Check sheet for the modelled part. Datum: model origin and axes. Units: mm. A direction names the side the tool comes from. Give positions to 0.01 mm unless a question says otherwise; leave off trailing zeros. Loops run counter-clockwise (first coordinate to the right, second up) from the corner with the lowest first, then second, coordinate; pieces in that order, holes last. Notation, with made-up numbers: (69.5, 33) - (122.5, 33) arc R23 ccw to (122.5, 61) - close; hole circle Ø9 at (52.25, 34). An arc over 180 degrees is marked (long way). Use one line per item in the form item = value.
from build123d import *

# Parameters (mm, degrees)
F0_R     = 2.25
F0_R_2   = 1
F1_DEPTH = 4


with BuildPart() as f1:
    # F0 (on Front) → F1 (new body)
    with BuildSketch(Plane.XZ):
        with BuildLine():
            ThreePointArc((0.754098, -10), (7.825165, -7.071068), (10.754098, 0))
            Line((10.754098, 0), (10.754098, 10))
            Line((10.754098, 10), (10.754098, 15))
            Line((10.754098, 15), (10.754098, 25))
            ThreePointArc((10.754098, 25), (9.289631, 28.535534), (5.754098, 30))
            ThreePointArc((5.754098, 30), (-1.31697, 27.071068), (-4.245902, 20))
            Line((-4.245902, 20), (-4.245902, 15))
            ThreePointArc((-4.245902, 15), (-5.710369, 11.464466), (-9.245902, 10))
            Line((-9.245902, 10), (-15.348779, 10))
            ThreePointArc((-15.348779, 10), (-25.348779, 0), (-15.348779, -10))
            Line((-15.348779, -10), (0, -10))
            Line((0, -10), (0.754098, -10))
        make_face()
        with Locations((-15.348779, 0)):
            Circle(F0_R, mode=Mode.SUBTRACT)
        Circle(F0_R, mode=Mode.SUBTRACT)
        with Locations((6.754098, 15)):
            Circle(F0_R_2, mode=Mode.SUBTRACT)
        with Locations((6.754098, 25)):
            Circle(F0_R_2, mode=Mode.SUBTRACT)
    extrude(amount=F1_DEPTH)


solid = f1.part
Item 1: Section check B-B on x = -0.5. Record the boundary of the cut face in (y, z).
Answer block:
outline = (-4, -10) - (0, -10) - (0, -2.19) - (-4, -2.19) - close; (-4, 2.19) - (0, 2.19) - (0, 27.8) - (-4, 27.8) - close
Item 2: Gauge pin test, flat ends, axial feed: P1, Ø1.6, axis at x = 6.75, z = 15, coming from the +Y side; P2, Ø2.5, axis at x = 6.75, z = 25, coming from the +Y side; P3, Ø1.2, axis at x = -11, y = -2, coming from the +Z side. Record the tip position at first contact, or that the pin passes through.
Answer block:
P1 = through
P2 = 0
P3 = 10
Item 3: Thickness scan on L1, parallel to X at y = -0.9, z = 17; L2, parallel to Z at x = -12.5, y = -0.4; L3, parallel to Z at x = 6.5, y = -2.9. Record the ranges inside material, lowest first.
Answer block:
L1 = -4.25 to 10.75
L2 = -10 to 10
L3 = -8.18 to 14.03, 15.97 to 24.03, 25.97 to 29.94
Item 4: Access from +Z, -Z, +X, -X, +Y, -Y to the whole of each face (thin tool, end or side, straight path). Record for faces 5 (the face through (9.328, -1.972, 28.496)), 6 (the face through (-4.246, -2, 18)).
Answer block:
face_5 = +Z, +X, +Y, -Y
face_6 = +Z, -X, +Y, -Y
Item 5: Section check A-A on y = -1.35. Record the boundary of the cut face in (x, z), then the cut area to 3 significant figures.
Answer block:
outline = (-15.35, -10) - (0.75, -10) arc R10 ccw to (10.75, 0) - (10.75, 25) arc R5 ccw to (5.75, 30) arc R10 ccw to (-4.25, 20) - (-4.25, 15) arc R5 cw to (-9.25, 10) - (-15.35, 10) arc R10 ccw to start; hole circle Ø4.5 at (-15.35, 0); hole circle Ø4.5 at (0, 0); hole circle Ø2 at (6.75, 15); hole circle Ø2 at (6.75, 25)
area = 898 mm2
Item 6: Section check D-D on z = 19. Record the boundary of the cut face in (x, y).
Answer block:
outline = (-4.25, -4) - (10.75, -4) - (10.75, 0) - (-4.25, 0) - close
Item 7: Mould release check, pull along Z, two halves, no side actions. Record for faces 1 (the face through (-0.29, -1.97, 2.23)), 2 (the face through (-7, -2, -10)), 3 (the face through (-5.672, -1.972, 11.504)), 4 (the face through (-17.597, -1.972, 0.099)): released by +Z, released by -Z, zero draft, split by the parting line, or undercut.
Answer block:
face_1 = undercut
face_2 = released by -Z
face_3 = released by +Z
face_4 = undercut
Item 8: Section check C-C on z = 14.5. Record the boundary of the cut face in (x, y).
Answer block:
outline = (-4.27, -4) - (5.89, -4) - (5.89, 0) - (-4.27, 0) - close; (7.62, -4) - (10.75, -4) - (10.75, 0) - (7.62, 0) - close
